Work out the finished part from the listing and answer in its coordinate system (mm). Face numbers are marked on the shaded views. Coordinates: 2 decimals unless noted, no trailing zeros. Order: outer loops, then holes, each group sorted by start corner. A loop starts at its lowest first (then second) coordinate and runs counter-clockwise, first axis right, second up. Notation, with made-up numbers: (81, 78.5) -> (133, 78.5) arc R32 cw to (133, 115.5) -> close; hole circle Ø10 at (65.25, 23.5). An arc over 180 degrees is marked (long way). Use one line per item in the form item = value.
Autodesk Inventor part; units mm, degrees
ref_plane "YZ Plane" through (0, 0, 0) normal (1, 0, 0) x (0, 1, 0)
ref_plane "XZ Plane" through (0, 0, 0) normal (0, 1, 0) x (-1, 0, 0)
ref_plane "XY Plane" through (0, 0, 0) normal (0, 0, 1) x (1, 0, 0)
sketch "Sketch1" plane through (0, 0, 0) normal (0, 0, 1) x (1, 0, 0)
  circle A0 centre (0, 0) radius 3.175
  circle A1 centre (0, 0) radius 6.35
  circle A2 centre (0, 0) radius 3.9688
  dimension "d0" = 6.35
  dimension "d1" = 12.7
  dimension "d4" = 7.9375
extrude "Extrusion1" add sketch "Sketch1" along normal blind 3.175 contours A1 | A2
extrude "Extrusion2" add sketch "Sketch1" against normal blind 0.3969 contours A2
properties part number "Plastic Gear Bushing"
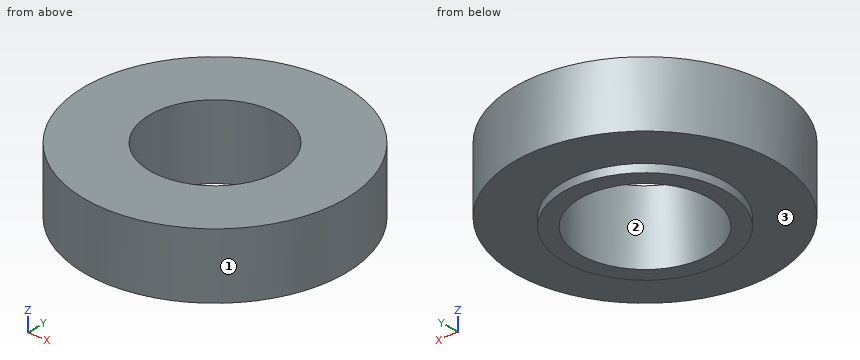
(1) Section A-A on x = 0 is taken. Write down the section's boundary in (y, z) (3 decimals), plus the area to 3 significant figures.
Data:
outline = (-6.35, 0) -> (-3.969, 0) -> (-3.969, -0.397) -> (-3.175, -0.397) -> (-3.175, 3.175) -> (-6.35, 3.175) -> close; (3.175, -0.397) -> (3.969, -0.397) -> (3.969, 0) -> (6.35, 0) -> (6.35, 3.175) -> (3.175, 3.175) -> close
area = 20.8 mm²
(2) Section D-D on y = 3.5 is taken. Write down the section's boundary in (x, z) (3 decimals), plus the area to 3 significant figures.
Data:
outline = (-5.298, 0) -> (-1.871, 0) -> (-1.871, -0.397) -> (1.871, -0.397) -> (1.871, 0) -> (5.298, 0) -> (5.298, 3.175) -> (-5.298, 3.175) -> close
area = 35.1 mm²
(3) Section C-C on z = 2.3 is taken. Write down the section's boundary in (x, y) (3 decimals).
Data:
outline = circle Ø12.7 at (0, 0); hole circle Ø6.35 at (0, 0)
(4) Straight lines are drawn through the part: line 1 along Y through (x, z) = (0, 1.9) (3 decimals); line 2 along Z through (x, y) = (2.5, -4.5) (3 decimals); line 3 along X through (y, z) = (1.25, -0.2). For each, find the intervals that lie inside material, in ascending order.
Data:
line_1 = -6.35 to -3.175, 3.175 to 6.35
line_2 = 0 to 3.175
line_3 = -3.77 to -2.92, 2.92 to 3.77
(5) Each of these flat-tipped pins is pushed along its axis until it touches: P1, Ø2, axis at y = 2.5, z = 0.5, coming from the +X side; P2, Ø1.5, axis at x = 4, y = -4.5, coming from the -Z side; P3, Ø5.5, axis at x = 0, y = 0, coming from the +Z side. Where does it stop, or does it pass through?
Data:
P1 = 6.17
P2 = 0
P3 = through
(6) The mould has two halves that part along X. Classify the marked faces 1, 2 and 3: released by +X, released by -X, zero draft, split by the parting line, or undercut.
Data:
face_1 = split by the parting line
face_2 = undercut
face_3 = zero draft
